Could you check a few things on this model? Use its own coordinates, in mm. A direction names the side the tool comes from. Coordinates: 2 decimals unless noted, no trailing zeros. Loops run counter-clockwise (first coordinate to the right, second up) from the corner with the lowest first, then second, coordinate; pieces in that order, holes last.
1) If I drill on line 1 along Z through (x, y) = (-172, 174); line 2 along X through (y, z) = (-2.5, 16.5); line 3 along Y through (x, z) = (102.5, 67.5), over which ranges is the centre line in solid material (lowest first)?
2) For faces 1 (the face through (221, -73, 90)), 2 (the face through (-249.76, 10.99, 4.93)), which set-ups out of +Z, -Z, +X, -X, +Y, -Y let a thin tool reach every point of the face, with its end or its side?
3) Imagine slicing it at C-C on z = 40. Please give me the cut outline in (x, y), plus the area to 3 significant figures.
4) Imagine slicing it at A-A on x = 0. Please give me the cut outline in (y, z).
5) Thinking about a two-plate mould opening in Z: for faces 3 (the face through (221, -73, 10)), 4 (the face through (-3, 4, 0)), 5 (the face through (-49.86, -224.53, 49.47)), 6 (the face through (-249.76, 10.99, 94.93)), which applies, released by +Z, released by -Z, zero draft, split by the parting line, or undercut?
6) Will these pins go through, and if not, where does the flat tip stop? P1, Ø12, axis at y = -6, z = 30, coming from the -X side; P2, Ø3, axis at x = -81.5, z = 82, coming from the -Y side; P3, Ø5, axis at x = 120, y = -49.5, coming from the -Z side; P4, Ø12, axis at x = -67, z = 48, coming from the -Y side.
```python
from build123d import *

# Parameters (mm, degrees)
F0_R     = 250
F1_DEPTH = 10
F2_R     = 230
F3_DEPTH = 80
F4_R     = 250
F5_DEPTH = 10
F6_R     = 2


with BuildPart() as f1:
    # F0 (on Top) → F1 (new body)
    with BuildSketch(Plane.XY):
        Circle(F0_R)
    extrude(amount=F1_DEPTH)

    # F2 (on face) → F3 (join)
    with BuildSketch(Plane.XY.offset(10)):
        Circle(F2_R)
    extrude(amount=F3_DEPTH)

    # F4 (on face) → F5 (join)
    with BuildSketch(Plane.XY.offset(90)):
        Circle(F4_R)
    extrude(amount=F5_DEPTH)

    # F6
    f6_edges = [f1.edges().sort_by_distance(p)[0] for p in [
        (230, 0, 50),
        (-230, 0, 10),
        (-230, 0, 90),
    ]]
    fillet(f6_edges, radius=F6_R)


solid = f1.part
```
Filled in:
1. line 1: z = 0 to 10, 90 to 100
1. line 2: x = -229.99 to 229.99
1. line 3: y = -205.9 to 205.9
2. face 1: none
2. face 2: +Z, -Z
3. outline: circle Ø460 at (0, 0)
3. area: 166,000 mm2
4. outline: (-250, 0) - (250, 0) - (250, 10) - (232, 10) arc R2 cw to (230, 12) - (230, 88) arc R2 cw to (232, 90) - (250, 90) - (250, 100) - (-250, 100) - (-250, 90) - (-232, 90) arc R2 cw to (-230, 88) - (-230, 12) arc R2 cw to (-232, 10) - (-250, 10) - close
5. face 3: undercut
5. face 4: released by -Z
5. face 5: undercut
5. face 6: zero draft
6. P1: stops at x = -230
6. P2: stops at y = -215.64
6. P3: stops at z = 0
6. P4: stops at y = -221.76
